Geometry: final body of the model. Coordinates: model frame, mm. Face numbers are marked on the shaded views. A direction names the side the tool comes from. Give positions to 0.01 mm unless a question says otherwise; leave off trailing zeros. Loops run counter-clockwise (first coordinate to the right, second up) from the corner with the lowest first, then second, coordinate; pieces in that order, holes last. Notation, with made-up numbers: (-29, 10) -> (8, 10) arc R35 ccw to (8, 47) -> close; hole circle Ø8 at (68.25, -4). An arc over 180 degrees is marked (long way). One line per question, with ' | ' between items. Start each with the question number.
Item 1: Material intervals for line 1 along Y through (x, z) = (0, 34); line 2 along Y through (x, z) = (-2.5, 1.75); line 3 along Z through (x, y) = (3.25, -3.75), sorted ascending. Write a range as [from, to].
Item 2: Section A-A on x = 0. Return loops of the section in (y, z).
Item 3: Section B-B on z = 32. Return loops of the section in (x, y).
Item 4: Pin query (flat end, axial travel): P1, Ø0.6, axis at x = 2, y = 0, coming from the -Z side; P2, Ø0.6, axis at x = -2, y = 8, coming from the -Z side; P3, Ø1.5, axis at x = 5.5, y = -6.5, coming from the +Z side. Return the tip coordinate at first contact, or that it passes through.
Item 5: Set-up query: the marked faces 1, 2, 3, 4 and 5. Return all of +Z, -Z, +X, -X, +Y, -Y with unobstructed straight access to the full face (end or side cutting, diameter ignored); none if empty.
Item 6: Mould query, pull axis X, two halves, no side actions, for the marked faces 6, 7 and 8. Classes: released by +X, released by -X, zero draft, split by the parting line, or undercut.
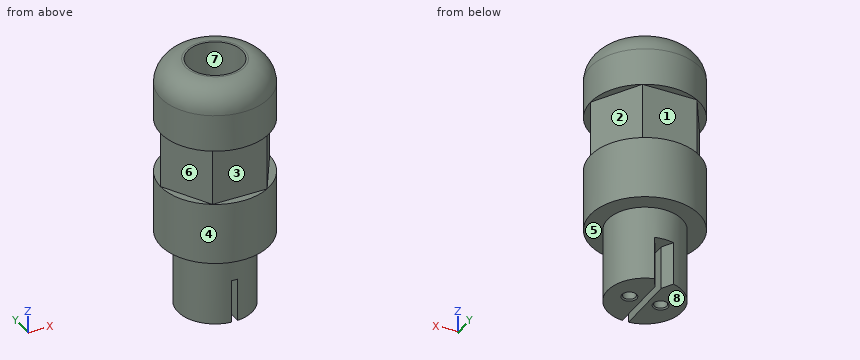
from build123d import *

# Parameters (mm, degrees)
SKETCH1_R           = 6
BOSS_EXTRUDE1_DEPTH = 12
SKETCH2_R           = 8.75
BOSS_EXTRUDE2_DEPTH = 10
BOSS_EXTRUDE3_DEPTH = 9
SKETCH4_R           = 8.75
BOSS_EXTRUDE4_DEPTH = 10
FILLET1_R           = 4
SKETCH5_R           = 4.4
CUT_EXTRUDE1_DEPTH  = 20
CUT_EXTRUDE2_DEPTH  = 7
SKETCH7_R           = 1
CUT_EXTRUDE3_DEPTH  = 7
CHAMFER1_SIZE       = 0.2


with BuildPart() as part:
    # Sketch1 → Boss-Extrude1 (new body)
    with BuildSketch(Plane.XY):
        Circle(SKETCH1_R)
    extrude(amount=BOSS_EXTRUDE1_DEPTH)

    # Sketch2 → Boss-Extrude2 (add)
    with BuildSketch(Plane.XY.offset(12)):
        Circle(SKETCH2_R)
    extrude(amount=BOSS_EXTRUDE2_DEPTH)

    # Sketch3 → Boss-Extrude3 (add)
    with BuildSketch(Plane.XY.offset(22)):
        Polygon((4.375, 7.577722283), (-4.375, 7.577722283), (-8.75, 0), (-4.375, -7.577722283), (4.375, -7.577722283), (8.75, 0), align=None)
    extrude(amount=BOSS_EXTRUDE3_DEPTH)

    # Sketch4 → Boss-Extrude4 (add)
    with BuildSketch(Plane.XY.offset(31)):
        Circle(SKETCH4_R)
    extrude(amount=BOSS_EXTRUDE4_DEPTH)

    # Fillet1
    fillet1_edges = [part.edges().sort_by_distance(p)[0] for p in [
        (-8.75, 0, 41),
    ]]
    fillet(fillet1_edges, radius=FILLET1_R)

    # Sketch5 → Cut-Extrude1 (cut)
    with BuildSketch(Plane.XY.offset(41)):
        Circle(SKETCH5_R)
    extrude(amount=-CUT_EXTRUDE1_DEPTH, mode=Mode.SUBTRACT)

    # Sketch6 → Cut-Extrude2 (cut)
    with BuildSketch(Plane(origin=(0, 0, 0), x_dir=(-1, 0, 0), z_dir=(0, 0, -1))):
        with BuildLine():
            Line((-0.5, -5.979130372), (-0.5, 4))
            Line((-0.5, 4), (-1.538832081, 5.799309944))
            ThreePointArc((-1.538832081, 5.799309944), (0, 6), (1.538832081, 5.799309944))
            Line((1.538832081, 5.799309944), (0.5, 4))
            Line((0.5, 4), (0.5, -5.979130372))
            ThreePointArc((0.5, -5.979130372), (0, -6), (-0.5, -5.979130372))
        make_face()
    extrude(amount=-CUT_EXTRUDE2_DEPTH, mode=Mode.SUBTRACT)

    # Sketch7 → Cut-Extrude3 (cut)
    with BuildSketch(Plane(origin=(0, 0, 0), x_dir=(-1, 0, 0), z_dir=(0, 0, -1))):
        with Locations((-2.5, 0)):
            Circle(SKETCH7_R)
        with Locations((2.5, 0)):
            Circle(SKETCH7_R)
    extrude(amount=-CUT_EXTRUDE3_DEPTH, mode=Mode.SUBTRACT)

    # Chamfer1
    chamfer1_edges = [part.edges().sort_by_distance(p)[0] for p in [
        (3.5, 0, 0),
        (-1.5, 0, 0),
    ]]
    chamfer(chamfer1_edges, length=CHAMFER1_SIZE)


solid = part.part
Result sheet:
1) line 1: y = [-8.75, -4.4], [4.4, 8.75] | line 2: y = [-5.45, -1], [1, 5.45] | line 3: z = [0, 40.99]
2) outline: (-8.75, 12) -> (-6, 12) -> (-6, 7) -> (6, 7) -> (6, 12) -> (8.75, 12) -> (8.75, 22) -> (7.58, 22) -> (7.58, 31) -> (8.75, 31) -> (8.75, 37) arc R4 ccw to (4.75, 41) -> (4.4, 41) -> (4.4, 21) -> (-4.4, 21) -> (-4.4, 41) -> (-4.75, 41) arc R4 ccw to (-8.75, 37) -> (-8.75, 31) -> (-7.58, 31) -> (-7.58, 22) -> (-8.75, 22) -> close
3) outline: circle Ø17.5 at (0, 0); hole circle Ø8.8 at (0, 0)
4) P1: stops at z = 7 | P2: stops at z = 12 | P3: stops at z = 39.63
5) face 1: +X, -X, +Y | face 2: +X, +Y | face 3: +X, -X, -Y | face 4: +Z, -Z | face 5: -Z
6) face 6: released by -X | face 7: undercut | face 8: zero draft
